Could you check a few things on this drawing? It's one solid part, dimensions in mm from its lowest x, y, z. A direction names the side the tool comes from. Round coordinates to 2 decimals unless told otherwise and drop trailing zeros. Order: outer loops, then holes, each group sorted by start corner. A loop starts at its lowest first (then second) coordinate and runs counter-clockwise, first axis right, second up. Notation, with made-up numbers: M 25,41.25 L 32,41.25 A16 ccw 32,53.25 Z; hole C 39.25,-9 d8. An arc over 180 degrees is marked long. Answer as CSV lines item,"result". Start each with the question number.
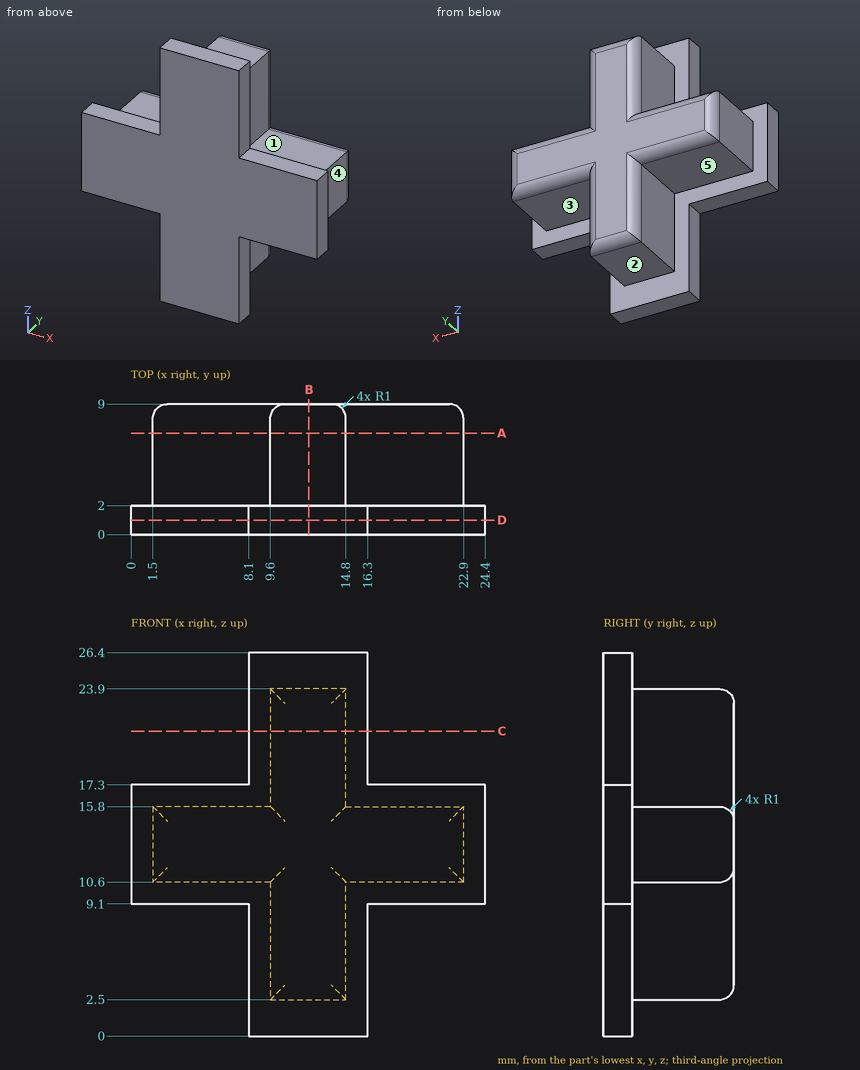
Item 1: For P1, Ø0.6, axis at y = 0.5, z = 24, coming from the +X side; P2, Ø2, axis at x = 5.5, y = 1, coming from the -Z side; P3, Ø1, axis at x = 20, z = 16, coming from the +Y side, each with a flat end and sliding along its axis, tell me the tip position at first contact or that it passes through.
Item 2: If we section it at A-A on y = 7: Please give me the cut outline in (x, z), and give its area (3 significant figures).
Item 3: If we section it at B-B on x = 12.25: Please give me the cut outline in (y, z), and give its area (3 significant figures).
Item 4: Which directions (+Z, -Z, +X, -X, +Y, -Y) give clear straight access to the entire face, cutting with the end or side of a thin tool? Please do the marked faces 1, 2, 3, 4 and 5.
Item 5: If we section it at D-D on y = 1: Please give me the cut outline in (x, z), and give its area (3 significant figures).
Item 6: If we section it at C-C on z = 21: Please give me the cut outline in (x, y).
Item 7: If I drill on line 1 along Y through (x, z) = (6.25, 17); line 2 along X through (y, z) = (7, 3.75); line 3 along Z through (x, y) = (22.75, 3.25), over which ranges is the centre line in solid material (lowest first)?
Geometry says:
1,P1,"x = 16.3"
1,P2,"z = 9.1"
1,P3,"y = 8.71"
2,outline,"M 1.5,10.6 L 9.6,10.6 L 9.6,2.5 L 14.8,2.5 L 14.8,10.6 L 22.9,10.6 L 22.9,15.8 L 14.8,15.8 L 14.8,23.9 L 9.6,23.9 L 9.6,15.8 L 1.5,15.8 Z"
2,area,"196 mm²"
3,outline,"M 0,0 L 2,0 L 2,2.5 L 8,2.5 A1 ccw 9,3.5 L 9,22.9 A1 ccw 8,23.9 L 2,23.9 L 2,26.4 L 0,26.4 Z"
3,area,"202 mm²"
4,face 1,"+Z, +X, +Y"
4,face 2,"-Z, +X, -X, +Y"
4,face 3,"-Z, +X, +Y"
4,face 4,"+Z, -Z, +X, +Y"
4,face 5,"-Z, -X, +Y"
5,outline,"M 0,9.1 L 8.1,9.1 L 8.1,0 L 16.3,0 L 16.3,9.1 L 24.4,9.1 L 24.4,17.3 L 16.3,17.3 L 16.3,26.4 L 8.1,26.4 L 8.1,17.3 L 0,17.3 Z"
5,area,"349 mm²"
6,outline,"M 8.1,0 L 16.3,0 L 16.3,2 L 14.8,2 L 14.8,8 A1 ccw 13.8,9 L 10.6,9 A1 ccw 9.6,8 L 9.6,2 L 8.1,2 Z"
7,line 1,"0 to 2"
7,line 2,"9.6 to 14.8"
7,line 3,"10.6 to 15.8"
